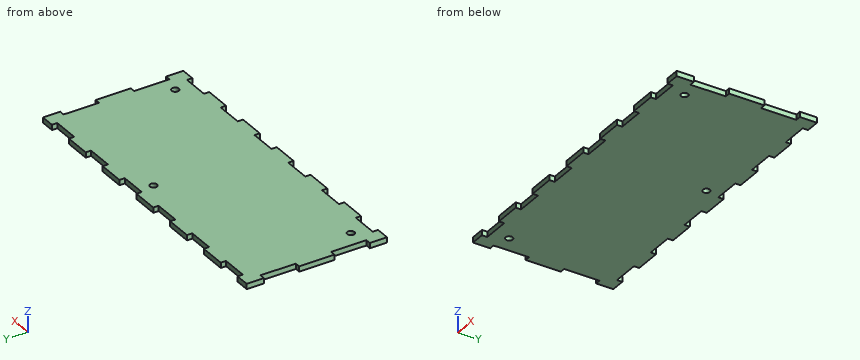
Autodesk Inventor part; units mm, degrees
ref_plane "YZ Plane" through (0, 0, 0) normal (1, 0, 0) x (0, 1, 0)
ref_plane "XZ Plane" through (0, 0, 0) normal (0, 1, 0) x (-1, 0, 0)
ref_plane "XY Plane" through (0, 0, 0) normal (0, 0, 1) x (1, 0, 0)
sketch "Sketch1" plane through (0, 0, 0) normal (0, 0, 1) x (1, 0, 0)
  line L0 (-87.5, -36.75) -> (87.5, -36.75)
  line L1 (87.5, -36.75) -> (87.5, 36.75)
  line L2 (87.5, 36.75) -> (-87.5, 36.75)
  line L3 (-87.5, 36.75) -> (-87.5, -36.75)
  line L4 (-87.5, -36.75) -> (87.5, 36.75) construction
  line L5 (87.5, -36.75) -> (-87.5, 36.75) construction
  line L6 (-67.5, 36.75) -> (-52.5, 36.75)
  line L7 (-52.5, 36.75) -> (-52.5, 39.75)
  line L8 (-52.5, 39.75) -> (-67.5, 39.75)
  line L9 (-67.5, 39.75) -> (-67.5, 36.75)
  line L10 (-87.5, 10) -> (-90.5, 10)
  line L11 (-90.5, 10) -> (-90.5, -10)
  line L12 (-90.5, -10) -> (-87.5, -10)
  line L13 (-87.5, -10) -> (-87.5, 10)
  line L14 (-82.5, 36.75) -> (-82.5, 39.75)
  line L15 (-87.5, 30) -> (-90.5, 30)
  line L16 (-90.5, 30) -> (-90.5, 39.75)
  line L17 (-90.5, 39.75) -> (-82.5, 39.75)
  line L18 (-22.5, 36.75) -> (-22.5, 39.75)
  line L19 (-22.5, 39.75) -> (-37.5, 39.75)
  line L20 (-37.5, 39.75) -> (-37.5, 36.75)
  line L21 (-37.5, 36.75) -> (-22.5, 36.75)
  line L22 (7.5, 36.75) -> (7.5, 39.75)
  line L23 (7.5, 39.75) -> (-7.5, 39.75)
  line L24 (-7.5, 39.75) -> (-7.5, 36.75)
  line L25 (-7.5, 36.75) -> (7.5, 36.75)
  line L26 (37.5, 36.75) -> (37.5, 39.75)
  line L27 (37.5, 39.75) -> (22.5, 39.75)
  line L28 (22.5, 39.75) -> (22.5, 36.75)
  line L29 (22.5, 36.75) -> (37.5, 36.75)
  line L30 (67.5, 36.75) -> (67.5, 39.75)
  line L31 (67.5, 39.75) -> (52.5, 39.75)
  line L32 (52.5, 39.75) -> (52.5, 36.75)
  line L33 (52.5, 36.75) -> (67.5, 36.75)
  line L34 (-52.5, -39.75) -> (-52.5, -36.75)
  line L35 (-52.5, -36.75) -> (-67.5, -36.75)
  line L36 (-67.5, -36.75) -> (-67.5, -39.75)
  line L37 (-67.5, -39.75) -> (-52.5, -39.75)
  line L38 (-22.5, -39.75) -> (-22.5, -36.75)
  line L39 (-22.5, -36.75) -> (-37.5, -36.75)
  line L40 (-37.5, -36.75) -> (-37.5, -39.75)
  line L41 (-37.5, -39.75) -> (-22.5, -39.75)
  line L42 (7.5, -39.75) -> (7.5, -36.75)
  line L43 (7.5, -36.75) -> (-7.5, -36.75)
  line L44 (-7.5, -36.75) -> (-7.5, -39.75)
  line L45 (-7.5, -39.75) -> (7.5, -39.75)
  line L46 (37.5, -39.75) -> (37.5, -36.75)
  line L47 (37.5, -36.75) -> (22.5, -36.75)
  line L48 (22.5, -36.75) -> (22.5, -39.75)
  line L49 (22.5, -39.75) -> (37.5, -39.75)
  line L50 (67.5, -39.75) -> (67.5, -36.75)
  line L51 (67.5, -36.75) -> (52.5, -36.75)
  line L52 (52.5, -36.75) -> (52.5, -39.75)
  line L53 (52.5, -39.75) -> (67.5, -39.75)
  line L54 (90.5, 10) -> (87.5, 10)
  line L55 (87.5, 10) -> (87.5, -10)
  line L56 (87.5, -10) -> (90.5, -10)
  line L57 (90.5, -10) -> (90.5, 10)
  line L58 (-87.5, 0) -> (87.5, 0) construction
  line L59 (0, 36.75) -> (0, -36.75) construction
  line L60 (-87.5, 30) -> (-87.5, 36.75)
  line L61 (-82.5, 36.75) -> (-87.5, 36.75)
  line L62 (-82.5, -36.75) -> (-82.5, -39.75)
  line L63 (-87.5, -30) -> (-90.5, -30)
  line L64 (-90.5, -30) -> (-90.5, -39.75)
  line L65 (-90.5, -39.75) -> (-82.5, -39.75)
  line L66 (-87.5, -30) -> (-87.5, -36.75)
  line L67 (-82.5, -36.75) -> (-87.5, -36.75)
  line L68 (82.5, 36.75) -> (82.5, 39.75)
  line L69 (87.5, 30) -> (90.5, 30)
  line L70 (90.5, 30) -> (90.5, 39.75)
  line L71 (90.5, 39.75) -> (82.5, 39.75)
  line L72 (87.5, 30) -> (87.5, 36.75)
  line L73 (82.5, 36.75) -> (87.5, 36.75)
  line L74 (82.5, -36.75) -> (82.5, -39.75)
  line L75 (87.5, -30) -> (90.5, -30)
  line L76 (90.5, -30) -> (90.5, -39.75)
  line L77 (90.5, -39.75) -> (82.5, -39.75)
  line L78 (87.5, -30) -> (87.5, -36.75)
  line L79 (82.5, -36.75) -> (87.5, -36.75)
  point P0 (0, 0)
  dimension "d0" = 175
  dimension "d1" = 73.5
  dimension "d2" = 15
  dimension "d3" = 3
  dimension "d4" = 20
  dimension "d5" = 3
  dimension "d6" = 20
  dimension "d7" = 10
  dimension "d8" = 3
  dimension "d9" = 15
  dimension "d10" = 3
  dimension "d11" = 20
  dimension "d14" = 30
  dimension "d17" = 76.5
  dimension "d22" = 178
extrude "Extrusion1" add sketch "Sketch1" along normal blind 3
sketch "Sketch2" plane through (0, 0, 3) normal (0, 0, 1) x (1, 0, 0)
  circle A0 centre (-78, -27.25) radius 2
  circle A1 centre (78, -27.25) radius 2
  line L0 (87.5, -30) -> (87.5, -10)
  line L1 (67.5, -36.75) -> (82.5, -36.75)
  line L2 (-82.5, -36.75) -> (-67.5, -36.75)
  line L3 (-87.5, -10) -> (-87.5, -30)
  point P0 (0, 0)
  dimension "d29" = 4
  dimension "d30" = 4
  dimension "d31" = 9.5
  dimension "d32" = 9.5
  dimension "d33" = 9.5
  dimension "d34" = 9.5
extrude "Extrusion2" cut sketch "Sketch2" against normal blind 10
sketch "Sketch3" plane through (0, 0, 0) normal (0, 0, -1) x (-1, 0, 0)
  circle A0 centre (-9.5, 28.75) radius 2
  line L0 (-7.5, 39.75) -> (-7.5, 36.75)
  line L1 (-22.5, 36.75) -> (-7.5, 36.75)
  point P0 (0, 0)
  dimension "d37" = 4
  dimension "d38" = 2
  dimension "d39" = 8
extrude "Extrusion3" cut sketch "Sketch3" against normal blind 10
equation "\"BendRadius\" = Thickness"
equation "\"BendReliefWidth\" = Thickness"
equation "\"BendReliefDepth\" = 0.5 * Thickness"
equation "\"CornerReliefSize\" = 4 * Thickness"
equation "\"MinimumRemnant\" = 2 * Thickness"
equation "\"TransitionRadius\" = BendRadius"
equation "\"JacobiRadiusSize\" = BendRadius"
equation "\"GapSize\" = Thickness"
properties part number "12 boven plaat LCD"
Can you work these out from the model? Positions are in its coordinate system, mm. Coordinates: 2 decimals unless noted, no trailing zeros. Write each loop counter-clockwise with the first axis right and the second up, starting at its lowest first coordinate (ties: lowest second). Pieces come first, ordered by that corner, then holes. Notation, with made-up numbers: (23, -24) - (57, -24) arc R34 ccw to (57, 14) - close; hole circle Ø6 at (11.25, -26). An arc over 180 degrees is marked (long way). Return JSON: item names as keys, results as strings. Group by question number.
Item 1: If we section it at C-C (z = 1.9): Count the separate pieces of the cut face and the enclosed holes in it, then the cut area to 3 significant figures.
Item 2: If we section it at B-B (y = -27.25): Write out the boundary of the cut face in (x, z), then the cut area to 3 significant figures.
Item 3: Please list where these lines run through material, in increasing order: probe 1 along Y at (x, z) = (-78, 1.15); probe 2 along Y at (x, z) = (9.5, 1.25); probe 3 along X at (y, z) = (14.5, 0.9).
Item 4: I'm going to push flat-ended pins straight in: pin 1 Ø0.9 at (y, z) = (-16, 2) entering from +X; pin 2 Ø0.9 at (x, z) = (-13, 2) entering from -Y. Where does each tip first touch, or does it pass through?
Item 5: If we section it at A-A (x = 9.5): Write out the boundary of the cut face in (y, z), then the cut area to 4 significant figures.
Return value:
{
 "1": {"separate pieces": "1", "enclosed holes": "3", "area": "13,600 mm^2"},
 "2": {"outline": "(-87.5, 0) - (-80, 0) - (-80, 3) - (-87.5, 3) - close; (-76, 0) - (76, 0) - (76, 3) - (-76, 3) - close; (80, 0) - (87.5, 0) - (87.5, 3) - (80, 3) - close", "area": "501 mm^2"},
 "3": {"probe 1": "y = -36.75 to -29.25, -25.25 to 36.75", "probe 2": "y = -36.75 to 26.75, 30.75 to 36.75", "probe 3": "x = -87.5 to 87.5"},
 "4": {"pin 1": "stops at x = 87.5", "pin 2": "stops at y = -36.75"},
 "5": {"outline": "(-36.75, 0) - (26.75, 0) - (26.75, 3) - (-36.75, 3) - close; (30.75, 0) - (36.75, 0) - (36.75, 3) - (30.75, 3) - close", "area": "208.5 mm^2"}
}
